Here's the drawing with two shaded views (mm, measured from the low corner). I have some questions. A direction names the side the tool comes from. Give positions to 0.01 mm unless a question says otherwise; leave off trailing zeros. Loops run counter-clockwise (first coordinate to the right, second up) from the corner with the lowest first, then second, coordinate; pieces in that order, holes last. Notation, with made-up numbers: M 89,81 L 124,81 A26 ccw 124,112 Z; hole C 7.5,31 d7. An arc over 180 degrees is marked long. Write item = value, one per line. Start each with the question number.
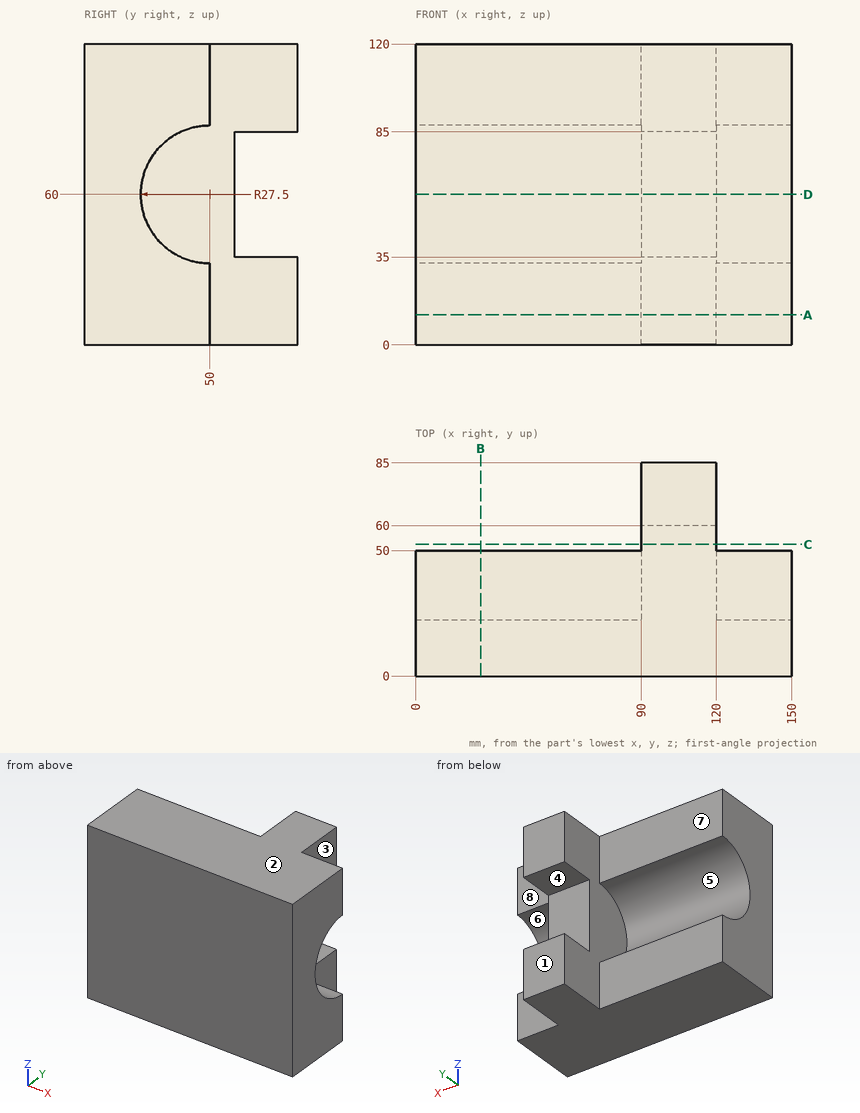
Q1. On a 3-axis mill with a long thin cutter (end or side, diameter ignored), from which of +Z, -Z, +X, -X, +Y, -Y can I reach the whole of each face in a straight line? I mean the marked faces 4, 5, 6, 7 and 8. Say none if no direction works.
Q2. If we section it at C-C, the plane y = 52.5: List the corners of the cut face in (x, z) for me, then the cut area to 3 significant figures.
Q3. Will these pins go through, and if not, where does the flat tip stop? pin 1 (3 mm diameter, centred on y = 32, z = 56.5, fed in from -X); pin 2 (9 mm diameter, centred on x = 128.5, z = 22.5, fed in from +Y); pin 3 (10 mm diameter, centred on x = 123, z = 75.5, fed in from +Y).
Q4. If we section it at A-A, the plane z = 12: List the corners of the cut face in (x, y) for me, then the cut area to 3 significant figures.
Q5. If we section it at B-B, the plane x = 26: List the corners of the cut face in (y, z) for me, then the cut area to 3 significant figures.
Q6. If we section it at D-D, the plane z = 60: List the corners of the cut face in (x, y) for me, then the cut area to 3 significant figures.
Q7. If I drill on line 1 along Z through (x, y) = (100, 77.5); line 2 along Y through (x, z) = (29, 106); line 3 along X through (y, z) = (56.5, 13.5), over which ranges is the centre line in solid material (lowest first)?
Q8. We'd pull the mould along Z, two halves only. Please class the marked faces 1, 2 and 3: pulls with the +Z half, pulls with the -Z half, needs draft (parallel to the pull), parting line crosses it, or undercut.
Resolved:
q1.face_4 = +X, -X, +Y
q1.face_5 = -X, +Y
q1.face_6 = +X, +Y
q1.face_7 = +Z, -Z, -X, +Y
q1.face_8 = +Z, -Z, +X, +Y
q2.outline = M 90,0 L 120,0 L 120,120 L 90,120 Z
q2.area = 3,600 mm²
q3.pin_1 = 90
q3.pin_2 = 50
q3.pin_3 = 60
q4.outline = M 0,0 L 150,0 L 150,50 L 120,50 L 120,85 L 90,85 L 90,50 L 0,50 Z
q4.area = 8,550 mm²
q5.outline = M 0,0 L 50,0 L 50,32.5 A27.5 cw 50,87.5 L 50,120 L 0,120 Z
q5.area = 4,810 mm²
q6.outline = M 0,0 L 150,0 L 150,22.5 L 120,22.5 L 120,60 L 90,60 L 90,22.5 L 0,22.5 Z
q6.area = 4,500 mm²
q7.line_1 = 0 to 35, 85 to 120
q7.line_2 = 0 to 50
q7.line_3 = 90 to 120
q8.face_1 = needs draft
q8.face_2 = pulls with the +Z half
q8.face_3 = undercut
